```python
from build123d import *

# Parameters (mm, degrees)
F0_W     = 50
F0_H     = 29
F1_DEPTH = 5
F2_R     = 1.45
F3_DEPTH = 38.6


with BuildPart() as f1:
    # F0 (on Top) → F1 (new body)
    with BuildSketch(Plane.XY):
        Rectangle(F0_W, F0_H)
    extrude(amount=F1_DEPTH)

    # F2 (on face) → F3 (cut)
    with BuildSketch(Plane.XZ.offset(14.5)):
        with Locations((0, 2.5)):
            Circle(F2_R)
    extrude(amount=-F3_DEPTH, mode=Mode.SUBTRACT)


solid = f1.part
```
The listing builds one solid part. Answer for the finished solid, in the listing's coordinates (mm). Coordinates: 2 decimals unless noted, no trailing zeros. Write each loop counter-clockwise with the first axis right and the second up, starting at its lowest first coordinate (ties: lowest second). Pieces come first, ordered by that corner, then holes. Notation, with made-up numbers: (-14.75, -14) - (9.25, -14) arc R28 ccw to (9.25, 25) - close; hole circle Ø11 at (-16.75, -17.75). An arc over 180 degrees is marked (long way). Return JSON: item names as keys, results as strings. Group by question number.
Q1. For a pull along X with two mould halves and no side action, classify faces 1 (the flat face through (0, 0, 5)), 2 (the flat face through (25, 0, 2)), 3 (the cylindrical face through (-0.189, -0.203, 3.938)) as +X half, -X half, draft (parallel to the pull), parting line (faces both ways), or undercut.
Q2. Find the intervals of material crossed by line 1 along Z through (x, y) = (0, -4.5); line 2 along X through (y, z) = (-5.75, 2.45); line 3 along X through (y, z) = (10.75, 1.55), in increasing order. Write a range as [from, to].
Q3. The part is cut by section B-B on x = 0. Write down the section's boundary in (y, z).
Q4. The part is cut by section A-A on z = 2.5. Write down the section's boundary in (x, y).
Q5. The part is cut by section C-C on y = 8.5. Write down the section's boundary in (x, z).
Evaluation:
{
 "1": {"face 1": "draft", "face 2": "+X half", "face 3": "undercut"},
 "2": {"line 1": "z = [0, 1.05], [3.95, 5]", "line 2": "x = [-25, -1.45], [1.45, 25]", "line 3": "x = [-25, -1.1], [1.1, 25]"},
 "3": {"outline": "(-14.5, 0) - (14.5, 0) - (14.5, 1.05) - (-14.5, 1.05) - close; (-14.5, 3.95) - (14.5, 3.95) - (14.5, 5) - (-14.5, 5) - close"},
 "4": {"outline": "(-25, -14.5) - (-1.45, -14.5) - (-1.45, 14.5) - (-25, 14.5) - close; (1.45, -14.5) - (25, -14.5) - (25, 14.5) - (1.45, 14.5) - close"},
 "5": {"outline": "(-25, 0) - (25, 0) - (25, 5) - (-25, 5) - close; hole circle Ø2.9 at (0, 2.5)"}
}
